Autodesk Inventor part; units mm, degrees
ref_plane "YZ Plane" through (0, 0, 0) normal (1, 0, 0) x (0, 1, 0)
ref_plane "XZ Plane" through (0, 0, 0) normal (0, 1, 0) x (-1, 0, 0)
ref_plane "XY Plane" through (0, 0, 0) normal (0, 0, 1) x (1, 0, 0)
sketch "Sketch1" plane through (0, 0, 0) normal (0, 1, 0) x (-1, 0, 0)
  line L0 (-30, 50) -> (30, 50)
  line L1 (30, 50) -> (30, -50)
  line L2 (30, -50) -> (-30, -50)
  line L3 (-30, -50) -> (-30, 50)
  line L4 (-30, 50) -> (30, -50) construction
  line L5 (30, 50) -> (-30, -50) construction
  circle A0 centre (0, 8) radius 3
  circle A1 centre (20, -20) radius 3
  circle A2 centre (-20, -20) radius 3
  circle A3 centre (0, -20) radius 15
  point P0 (0, 0)
  dimension "d0" = 60
  dimension "d1" = 100
  dimension "d2" = 6
  dimension "d3" = 6
  dimension "d5" = 58
  dimension "d6" = 10
  dimension "d8" = 30
  dimension "d9" = 6
  dimension "d10" = 10
  dimension "d11" = 30
  dimension "d12" = 30
extrude "Extrusion1" add sketch "Sketch1" along normal blind 20
sketch "Sketch2" plane through (0, 0, 0) normal (0, -1, 0) x (1, 0, 0)
  line L0 (30, -50) -> (-30, -50)
  line L1 (7, -50) -> (7, 50)
  line L2 (-7, -50) -> (-7, 50)
  line L3 (30, 50) -> (30, -50)
  line L4 (-30, -50) -> (-30, 50)
  line L5 (7, -50) -> (30, -50)
  line L6 (30, 50) -> (30, -50)
  line L7 (30, 50) -> (7, 50)
  line L8 (-30, 50) -> (30, 50)
  line L9 (-7, -50) -> (-30, -50)
  line L10 (-30, -50) -> (-30, 50)
  line L11 (-30, 50) -> (-7, 50)
  point P0 (0, 0)
  dimension "d15" = 23
  dimension "d16" = 23
extrude "Extrusion2" add sketch "Sketch2" along normal blind 5 contours L0 L1 L7 L3 | L0 L4 L8 L2
sketch "Sketch3" plane through (0, -5, 0) normal (0, -1, 0) x (1, 0, 0)
  line L0 (30, -50) -> (-30, -50)
  line L1 (8, -50) -> (8, 50)
  line L2 (-30, 50) -> (30, 50)
  line L3 (-8, -50) -> (-8, 50)
  line L4 (30, -50) -> (30, 50)
  line L5 (-30, 50) -> (-30, -50)
  line L6 (8, -50) -> (30, -50)
  line L7 (30, 50) -> (30, -50)
  line L8 (30, 50) -> (8, 50)
  line L9 (-8, 50) -> (-30, 50)
  line L10 (-30, -50) -> (-8, -50)
  point P0 (0, 0)
  dimension "d19" = 22
  dimension "d20" = 22
extrude "Extrusion3" add sketch "Sketch3" along normal blind 10 contours L0 L1 L2 L4 | L0 L5 L2 L3
sketch "Sketch4" plane through (0, -15, 0) normal (0, -1, 0) x (1, 0, 0)
  line L0 (8, -50) -> (30, -50)
  line L1 (7, -50) -> (7, 50)
  line L2 (-30, 50) -> (30, 50)
  line L3 (-30, -50) -> (-8, -50)
  line L4 (30, -50) -> (30, 50)
  line L5 (-30, 50) -> (-30, -50)
  line L6 (7, -50) -> (30, -50)
  line L7 (30, 50) -> (30, -50)
  line L8 (30, 50) -> (7, 50)
  line L9 (-30, -50) -> (-30, 50)
  line L10 (-30, -50) -> (-30, 50)
  line L11 (-30, -50) -> (-7, -50)
  line L12 (-30, 50) -> (-7, 50)
  line L13 (-7, 50) -> (-7, -50)
  point P0 (0, 0)
  dimension "d23" = 23
  dimension "d25" = 23
  dimension "d26" = 100
extrude "Extrusion4" add sketch "Sketch4" along normal blind 5
sketch "Sketch5" plane through (0, -20, 0) normal (0, -1, 0) x (1, 0, 0)
  circle A0 centre (17, -35) radius 3
  circle A1 centre (17, 0) radius 3
  circle A2 centre (17, 35) radius 3
  circle A3 centre (-17, 35) radius 3
  circle A4 centre (-17, 0) radius 3
  circle A5 centre (-17, -35) radius 3
  line L0 (-7, 50) -> (-30, 50)
  line L1 (-30, 50) -> (-30, -50)
  line L2 (30, -50) -> (30, 50)
  point P0 (0, 0)
  dimension "d29" = 6
  dimension "d30" = 6
  dimension "d31" = 6
  dimension "d32" = 6
  dimension "d33" = 6
  dimension "d34" = 6
  dimension "d35" = 15
  dimension "d36" = 35
  dimension "d37" = 70
  dimension "d38" = 13
  dimension "d39" = 13
hole "Hole1" at (17, -20, -35) at (17, -20, 0) at (17, -20, 35) at (-17, -20, 35) at (-17, -20, 0) at (-17, -20, -35) direction (0, 1, 0) diameter 6 depth 9 tip angle 118
chamfer "Chamfer1" distance 2 angle 45 1 edges at (30, -20, 0) measured on face at (26.6594, -20, 0.1205)
chamfer "Chamfer2" distance 2 angle 45 1 edges at (-30, -20, 0) measured on face at (-26.6594, -20, -0.1205)
chamfer "Chamfer3" distance 2 angle 45 1 edges at (30, 20, 0) measured on face at (0.1205, 20, 36.9927)
chamfer "Chamfer4" distance 2 angle 45 1 edges at (-30, 20, 0) measured on face at (-0.7872, 20, 36.9927)
chamfer "Chamfer5" distance 2 angle 45 1 edges at (0, 20, -50) measured on face at (-0.1205, 20, 36.9927)
chamfer "Chamfer6" distance 2 angle 45 1 edges at (0, 20, 50) measured on face at (0.1205, 20, 36.9927)
sketch "Sketch6" plane through (7, 0, -50) normal (0, 0, -1) x (-1, 0, 0)
  circle A0 centre (17, 10) radius 4
  circle A1 centre (-3, 10) radius 4
  line L0 (37, -18) -> (37, 18)
  line L1 (-23, 18) -> (-23, -18)
  line L2 (35, 20) -> (-21, 20)
  point P0 (7, 0)
  dimension "d65" = 8
  dimension "d66" = 8
  dimension "d67" = 20
  dimension "d68" = 20
  dimension "d69" = 10
hole "Hole2" at (10, 10, -50) at (-10, 10, -50) direction (0, 0, 1) diameter 8 depth 12 tip angle 118
sketch "Sketch7" plane through (0, 20, 0) normal (0, 1, 0) x (1, 0, 0)
  point P0 (0, 0)
sketch "Sketch8" plane through (0, 0, 0) normal (0, -1, 0) x (1, 0, 0)
  line L0 (6.6295, 50) -> (7, 0)
  line L1 (7, -6.7335) -> (7, 50)
  line L2 (-7, 50) -> (-7, -6.7335)
  line L3 (-7, 0) -> (-7, 50)
  line L4 (-7, 50) -> (6.6295, 50)
  line L5 (-7, 50) -> (7, 50)
  line L6 (7, 0) -> (-7, 0)
  point P0 (0, 0)
extrude "Extrusion5" add sketch "Sketch8" along normal blind 0.01 contours L0 L6 L2 L4
sketch "Sketch9" plane through (0, 20, 0) normal (0, 1, 0) x (1, 0, 0)
  circle A0 centre (0, -8) radius 3
  line L0 (30, 50) -> (-30, 50)
  point P0 (0, 0)
  dimension "d79" = 6
  dimension "d80" = 58
hole "Hole3" at (0, 20, 8) direction (0, -1, 0) diameter 6 depth 10 tip angle 118
properties part number "Schneidführung"
Input: part model. Units: mm. Frame: model coordinates. A direction names the side the tool comes from. Give positions to 0.01 mm unless a question says otherwise; leave off trailing zeros. Order: outer loops, then holes, each group sorted by start corner. A loop starts at its lowest first (then second) coordinate and runs counter-clockwise, first axis right, second up.
1. Cut plane A-A (y = -16.5). Return loops of the section in (x, z), and give its area (3 significant figures).
Computed:
outline: (-30, -50) - (-7, -50) - (-7, 50) - (-30, 50) - close; (7, -50) - (30, -50) - (30, 50) - (7, 50) - close; hole circle Ø6 at (-17, -35); hole circle Ø6 at (-17, 0); hole circle Ø6 at (-17, 35); hole circle Ø6 at (17, -35); hole circle Ø6 at (17, 0); hole circle Ø6 at (17, 35)
area: 4,430 mm2
2. Draft query along Z for faces 6 (the face through (7, -17, -1)), 7 (the face through (9.577, 9.449, -36.014)), 8 (the face through (-20, 0, -20)), 9 (the face through (-10, 0, -20)). Return one class per face: released by +Z, released by -Z, zero draft, split by the parting line, or undercut.
Computed:
face 6: zero draft
face 7: released by -Z
face 8: undercut
face 9: undercut
3. Cut plane C-C (x = -21). Return loops of the section in (y, z), and give its area (3 significant figures).
Computed:
outline: (-20, -50) - (18, -50) - (20, -48) - (20, -22.83) - (0, -22.83) - (0, -17.17) - (20, -17.17) - (20, 48) - (18, 50) - (-20, 50) - close
area: 3,880 mm2
4. Set-up query: faces 1 (the face through (10, 0, -20)), 2 (the face through (-29, 19, 1)), 3 (the face through (7, -2, -1)), 4 (the face through (-30, 0, 1)), 5 (the face through (17, -15, -32)). Return all of +Z, -Z, +X, -X, +Y, -Y with unobstructed straight access to the full face (end or side cutting, diameter ignored); none if empty.
Computed:
face 1: +Y
face 2: +Z, -Z, -X, +Y
face 3: +Z, -Z, -Y
face 4: +Z, -Z, -X, +Y, -Y
face 5: -Y
5. Pin query (flat end, axial travel): pin 1 Ø4 at (x, z) = (12, -19) entering from +Y. Return the tip coordinate at first contact, or that it passes through.
Computed:
pin 1: stops at y = 0
6. Line query: probe 1 along Z at (x, y) = (0, 4.5); probe 2 along X at (y, z) = (10, -44.75); probe 3 along X at (y, z) = (-17, -35). Output: solid intervals per line, ascending.
Computed:
probe 1: z = -50 to -35, -5 to 5, 11 to 50
probe 2: x = -30 to -14, -6 to 6, 14 to 30
probe 3: x = -30 to -20, -14 to -7, 7 to 14, 20 to 30
